from build123d import *

# Parameters (mm, degrees)
SKETCH1_R           = 4.75
BOSS_EXTRUDE1_DEPTH = 3
BOSS_EXTRUDE3_DEPTH = 3
SKETCH4_W           = 11
SKETCH4_H           = 16.6
BOSS_EXTRUDE4_DEPTH = 3
SKETCH5_R           = 4
BOSS_EXTRUDE5_DEPTH = 3
FILLET6_R           = 5
FILLET7_R           = 1


with BuildPart() as part:
    # Sketch1 → Boss-Extrude1 (new body)
    with BuildSketch(Plane(origin=(0, 0, 0), x_dir=(1, 0, 0), z_dir=(0, 1, 0))):
        with BuildLine():
            Line((0, 26.15), (30, 26.15))
            ThreePointArc((30, 26.15), (53, 0), (30, -26.15))
            Line((30, -26.15), (0, -26.15))
            Line((0, -26.15), (0, 26.15))
        make_face()
        with Locations(Location((17.75, 13.4, 0), (0, 0, 270))):
            Circle(SKETCH1_R, mode=Mode.SUBTRACT)
        with Locations(Location((17.75, -13.4, 0), (0, 0, 270))):
            Circle(SKETCH1_R, mode=Mode.SUBTRACT)
        with Locations(Location((39.75, 0, 0), (0, 0, 270))):
            Circle(SKETCH1_R, mode=Mode.SUBTRACT)
    extrude(amount=BOSS_EXTRUDE1_DEPTH)

    # Sketch3 → Boss-Extrude3 (add)
    with BuildSketch(Plane.ZY):
        with BuildLine():
            Line((-8.3, 0), (8.3, 0))
            Line((8.3, 0), (21.3, 0))
            ThreePointArc((21.3, 0), (12.785306817, 3.118998966), (8.3, 11))
            Line((8.3, 11), (8.3, 62))
            Line((8.3, 62), (-8.3, 62))
            Line((-8.3, 62), (-8.3, 11))
            ThreePointArc((-8.3, 11), (-12.785306817, 3.118998966), (-21.3, 0))
            Line((-21.3, 0), (-8.3, 0))
        make_face()
    extrude(amount=BOSS_EXTRUDE3_DEPTH)

    # Sketch4 → Boss-Extrude4 (add)
    with BuildSketch(Plane(origin=(0, 62, 0), x_dir=(1, 0, 0), z_dir=(0, 1, 0))):
        with Locations((2.5, 0)):
            Rectangle(SKETCH4_W, SKETCH4_H)
    extrude(amount=BOSS_EXTRUDE4_DEPTH)

    # Sketch5 → Boss-Extrude5 (add)
    with BuildSketch(Plane.XY.offset(8.3)):
        with BuildLine():
            Line((0, 58), (0, 27))
            Line((0, 27), (-13, 27))
            ThreePointArc((-13, 27), (-28, 42.5), (-13, 58))
            Line((-13, 58), (0, 58))
        make_face()
        with Locations((-16, 42.5)):
            Circle(SKETCH5_R, mode=Mode.SUBTRACT)
    boss_extrude5 = extrude(amount=BOSS_EXTRUDE5_DEPTH)

    # Mirror1: Boss-Extrude5 across plane
    add(boss_extrude5.mirror(Plane.XY))

    # Fillet6
    # the kernel refuses this fillet: 5 mm, written as the material it takes off along each edge
    with BuildSketch(Plane(origin=(-3, 65, -20.8), x_dir=(0, -1, 0), z_dir=(0, 0, 1))) as fillet6_piece_1:
        with BuildLine():
            CenterArc((FILLET6_R, FILLET6_R), FILLET6_R, 180, 90)
            Line((0, FILLET6_R), (0, 0))
            Line((0, 0), (FILLET6_R, 0))
        make_face()
    extrude(amount=41.6, mode=Mode.SUBTRACT)
    with BuildSketch(Plane(origin=(-3, 0, 33.8), x_dir=(1, 0, 0), z_dir=(0, 0, -1))) as fillet6_piece_2:
        with BuildLine():
            CenterArc((FILLET6_R, -FILLET6_R), FILLET6_R, 90, 90)
            Line((0, -FILLET6_R), (0, 0))
            Line((0, 0), (FILLET6_R, 0))
        make_face()
    extrude(amount=67.6, mode=Mode.SUBTRACT)

    # Fillet7
    fillet7_edges = [part.edges().sort_by_distance(p)[0] for p in [
        (0, 3, 0),
    ]]
    fillet(fillet7_edges, radius=FILLET7_R)


solid = part.part
Could you check a few things on this model? Use its own coordinates, in mm. A direction names the side the tool comes from. Round coordinates to 2 decimals unless told otherwise and drop trailing zeros. Order: outer loops, then holes, each group sorted by start corner. A loop starts at its lowest first (then second) coordinate and runs counter-clockwise, first axis right, second up.
Q1. I'm going to push flat-ended pins straight in: P1, Ø12, axis at x = -16.5, y = 58.5, coming from the -Z side; P2, Ø0.9, axis at y = 63.5, z = 0, coming from the +X side; P3, Ø1.3, axis at y = 1.5, z = 19, coming from the -X side; P4, Ø2, axis at x = 4, y = 60, coming from the -Z side. Where does each tip first touch, or does it pass through?
Geometry says:
P1: stops at z = -11.3
P2: stops at x = 8
P3: stops at x = 0
P4: passes through
Q2. Which directions (+Z, -Z, +X, -X, +Y, -Y) give clear straight access to the entire face, cutting with the end or side of a thin tool? Please do faces 1 (the face through (-11, 43, -11.3)), 2 (the face through (-6, 27, -10)), 3 (the face through (0, 33, 0)), 4 (the face through (1.2, 62.2, 8.3)).
Geometry says:
face 1: -Z, +X, -X, +Y
face 2: -Z, +X, -X
face 3: +Z, -Z, +X
face 4: +Z, +X, -X, +Y
Q3. Imagine slicing it at B-B, the plane z = -3. List the corners of the cut face in (x, y) for me, then the cut area to 3 significant figures.
Geometry says:
outline: (-3, 5) arc R5 ccw to (2, 0) - (36.07, 0) - (36.07, 3) - (1, 3) arc R1 cw to (0, 4) - (0, 62) - (8, 62) - (8, 65) - (2, 65) arc R5 ccw to (-3, 60) - close; (43.43, 0) - (52.83, 0) - (52.83, 3) - (43.43, 3) - close
area: 345 mm2
Q4. Thinking about a two-plate mould opening in X: for faces 5 (the face through (-19.996, 42.676, -9.779)), 6 (the face through (-7, 58, -10)), 7 (the face through (-27.996, 42.166, 9.779)), which applies, released by +X, released by -X, zero draft, split by the parting line, or undercut?
Geometry says:
face 5: undercut
face 6: zero draft
face 7: released by -X
Q5. Imagine slicing it at A-A, the plane x = 17.75. List the corners of the cut face in (y, z) for me.
Geometry says:
outline: (0, -26.15) - (3, -26.15) - (3, -18.15) - (0, -18.15) - close; (0, -8.65) - (3, -8.65) - (3, 8.65) - (0, 8.65) - close; (0, 18.15) - (3, 18.15) - (3, 26.15) - (0, 26.15) - close
Q6. Imagine slicing it at D-D, the plane y = 33. List the corners of the cut face in (x, z) for me.
Geometry says:
outline: (-24.75, -11.3) - (0, -11.3) - (0, 11.3) - (-24.75, 11.3) - (-24.75, 8.3) - (-3, 8.3) - (-3, -8.3) - (-24.75, -8.3) - close
Q7. Imagine slicing it at C-C, the plane x = 39.75. List the corners of the cut face in (y, z) for me, then the cut area to 3 significant figures.
Geometry says:
outline: (0, -22.87) - (3, -22.87) - (3, -4.75) - (0, -4.75) - close; (0, 4.75) - (3, 4.75) - (3, 22.87) - (0, 22.87) - close
area: 109 mm2
Q8. Please list where these lines run through material, in increasing order: probe 1 along Z at (x, y) = (17, 2); probe 2 along Y at (x, z) = (40.5, -19.5); probe 3 along Y at (x, z) = (-16, -10).
Geometry says:
probe 1: z = -26.15 to -18.09, -8.71 to 8.71, 18.09 to 26.15
probe 2: y = 0 to 3
probe 3: y = 27.39 to 38.5, 46.5 to 57.61
